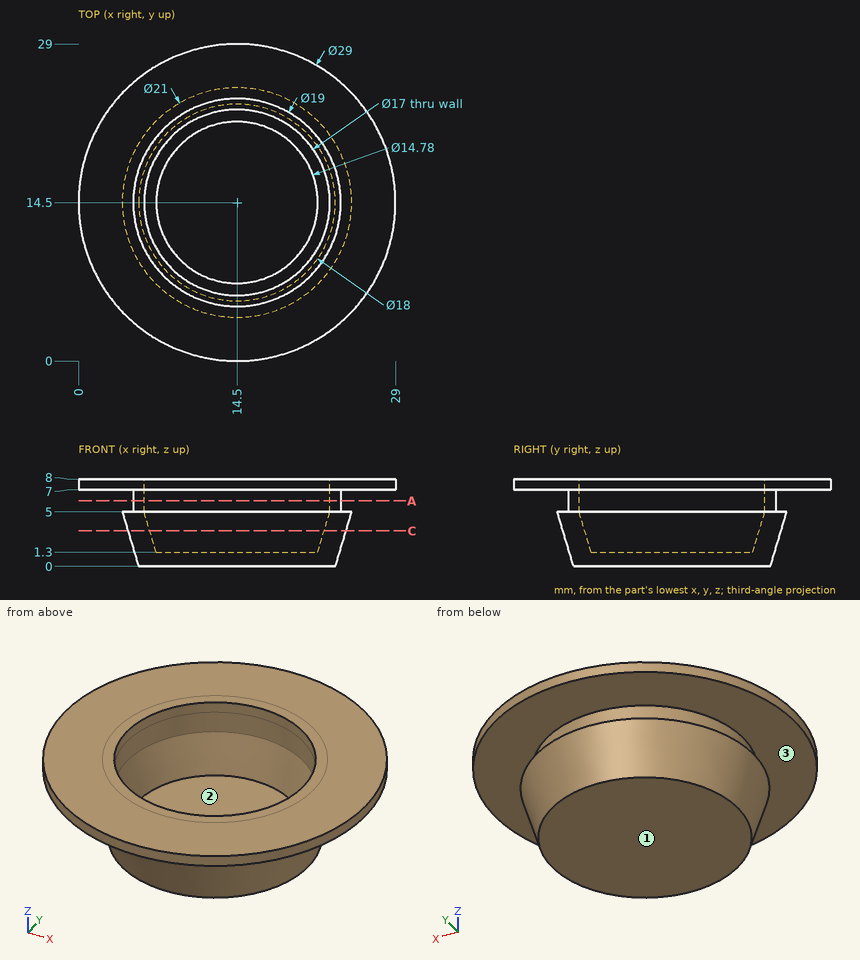
Job drawing, mm, ordinate dimensions from the low corner. One solid piece. Give positions to 0.01 mm unless a question says otherwise; leave off trailing zeros. Order: outer loops, then holes, each group sorted by start corner. A loop starts at its lowest first (then second) coordinate and runs counter-clockwise, first axis right, second up. Notation, with made-up numbers: M -7,3.5 L 39,3.5 A20 cw 39,15.5 Z; hole C 13,41.25 d10. An arc over 180 degrees is marked long. Put each result on its own line as item: value. Start each with the question number.
(1) Drill centre lines: L1, parallel to X at y = 14.5, z = 7.5; L2, parallel to Y at x = 14.5, z = 5.4. Where is each one in solid material? Low to high. Write a range as [from, to].
(2) Band-saw the part on A-A on z = 6. Give the cut face in (x, y).
(3) Pin check, flat tips, straight feed: pin 1 Ø4 at (y, z) = (8.5, 2.5) entering from +X; pin 2 Ø4 at (x, z) = (14, 1.5) entering from +Y; pin 3 Ø1.5 at (x, z) = (7, 3) entering from -Y. Stop position of each tip, or through.
(4) Band-saw the part on C-C on z = 3.25. Give the cut face in (x, y) (3 decimals).
(5) Pull direction Z, two halves, no side cores. Call the marked faces 1, 2 and 3: released by +Z, released by -Z, zero draft, split by the parting line, or undercut.
Results below:
1. L1: x = [0, 6], [23, 29]
1. L2: y = [5, 6], [23, 24]
2. outline: C 14.5,14.5 d19; hole C 14.5,14.5 d17
3. pin 1: stops at x = 23.6
3. pin 2: stops at y = 24.54
3. pin 3: stops at y = 7.19
4. outline: C 14.5,14.5 d19.95; hole C 14.5,14.5 d15.95
5. face 1: released by -Z
5. face 2: released by +Z
5. face 3: undercut
